Could you check a few things on this drawing? It's one solid part, dimensions in mm from its lowest x, y, z. Give positions to 0.01 mm unless a question says otherwise; leave off trailing zeros. Order: outer loops, then holes, each group sorted by start corner. A loop starts at its lowest first (then second) coordinate and runs counter-clockwise, first axis right, second up.
Item 1: If I drill on line 1 along X through (y, z) = (483.5, 1.25), over which ranges is the centre line in solid material (lowest first)?
Item 2: I want a section at B-B, the plane z = 3.5. Write out the boundary of the cut face in (x, y).
Item 3: I want a section at A-A, the plane y = 331.5. Write out the boundary of the cut face in (x, z), then the cut area to 3 significant figures.
Item 4: I'm going to push a flat-ended pin straight in: pin 1 Ø2 at (x, y) = (2, 180) entering from -Z. Where does the tip first touch, or does it pass through?
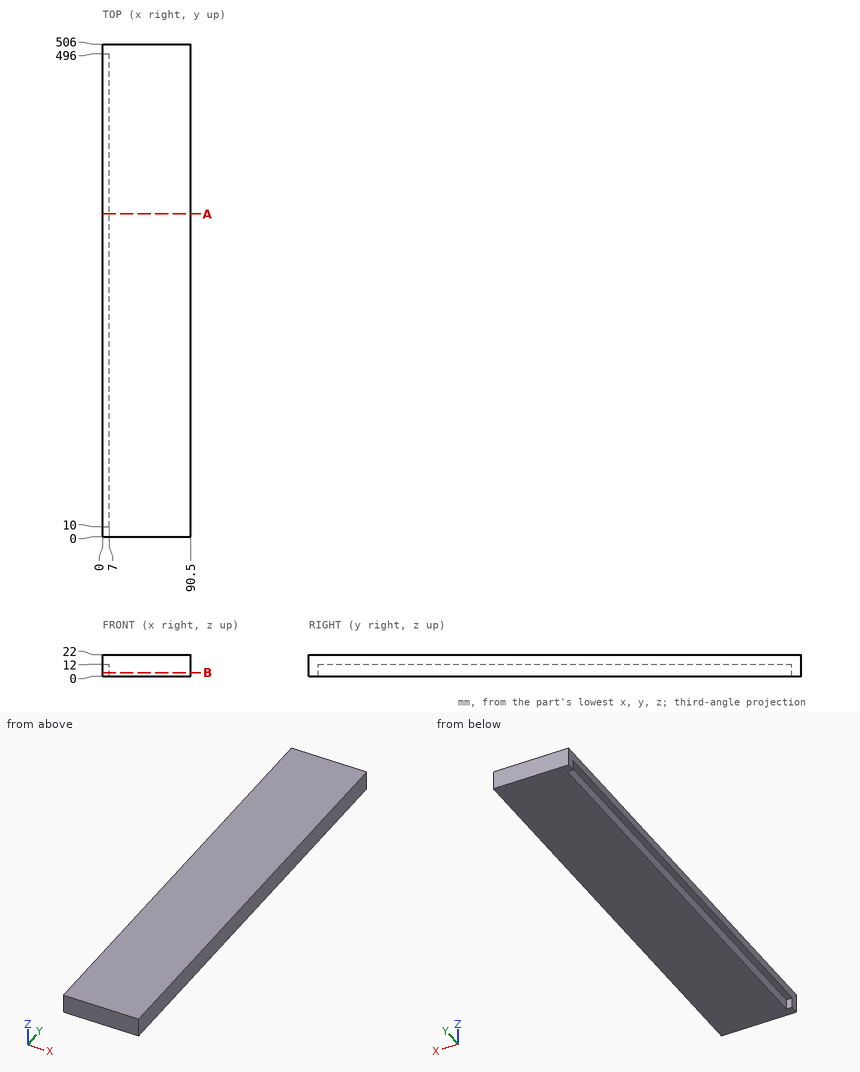
Results list:
1. line 1: x = 7 to 90.5
2. outline: (0, 0) - (90.5, 0) - (90.5, 506) - (0, 506) - (0, 496) - (7, 496) - (7, 10) - (0, 10) - close
3. outline: (0, 12) - (7, 12) - (7, 0) - (90.5, 0) - (90.5, 22) - (0, 22) - close
3. area: 1,910 mm2
4. pin 1: stops at z = 12
